Build history of the part. All positions in model axes, mm. Face numbers are marked on the shaded views. Coordinates: 2 decimals unless noted, no trailing zeros. Loops run counter-clockwise (first coordinate to the right, second up) from the corner with the lowest first, then second, coordinate; pieces in that order, holes last.
(1) Flat gauge pins, fed straight in: P1, Ø1, axis at x = -1, y = -1.5, coming from the -Z side; P2, Ø1.5, axis at y = 1, z = 2.5, coming from the +X side; P3, Ø0.7, axis at x = 0, z = -2, coming from the -Y side. Where does each tip first touch, or does it go through?
(2) Wall check: L1, parallel to Y at x = -0.75, z = 10.25; L2, parallel to X at y = 0.1, z = 15.5; L3, parallel to X at y = -1.3, z = 11. Give the ranges that are in metal, low to high.
(3) Two-plate mould, pull along X, no slides. Class the marked faces 1, 2 and 3: pulls with the +X half, pulls with the -X half, needs draft (parallel to the pull), parting line crosses it, or undercut.
(4) Slice it at A-A (z = 5.5). Give the cut face in (x, y).
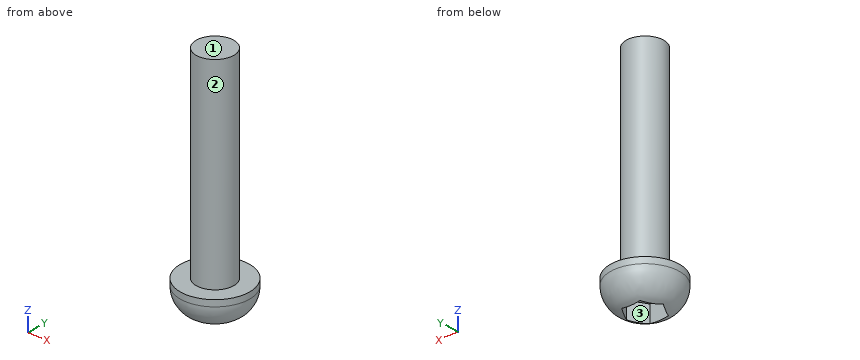
Autodesk Inventor part; units mm, degrees
ref_plane "YZ Plane" through (0, 0, 0) normal (1, 0, 0) x (0, 1, 0)
ref_plane "XZ Plane" through (0, 0, 0) normal (0, 1, 0) x (-1, 0, 0)
ref_plane "XY Plane" through (0, 0, 0) normal (0, 0, 1) x (1, 0, 0)
sketch "Boceto1" plane through (0, 0, 0) normal (0, 0, 1) x (1, 0, 0)
  circle A0 centre (0, 0) radius 1.5
  circle A1 centre (0, 0) radius 2.75
  dimension "d0" = 3
  dimension "d1" = 5.5
extrude "Extrusión1" add sketch "Boceto1" along normal blind 16 contours A0
extrude "Extrusión2" add sketch "Boceto1" against normal blind 2.5 contours A0 | A1
sketch "Boceto2" plane through (0, 0, -2.5) normal (0, 0, -1) x (-1, 0, 0)
  line L0 (1.5, 0) -> (0.75, -1.299)
  line L1 (0.75, -1.299) -> (-0.75, -1.299)
  line L2 (-0.75, -1.299) -> (-1.5, 0)
  line L3 (-1.5, 0) -> (-0.75, 1.299)
  line L4 (-0.75, 1.299) -> (0.75, 1.299)
  line L5 (0.75, 1.299) -> (1.5, 0)
  point P0 (0, 0)
  point P1 (0, 0)
  dimension "d6" = 3
fillet "Empalme1" radius 2 1 edges at (-2.75, 0, -2.5)
extrude "Extrusión4" cut sketch "Boceto2" against normal blind 1.5
thread "Rosca1"
properties part number "tonrilloM3x16mm" material "Acero inoxidable, 440C"
Response values:
1. P1: stops at z = -2.4
1. P2: stops at x = 1.48
1. P3: stops at y = -2.39
2. L1: y = -1.3 to 1.3
2. L2: x = -1.5 to 1.5
2. L3: x = -0.75 to 0.75
3. face 1: needs draft
3. face 2: parting line crosses it
3. face 3: undercut
4. outline: circle Ø3 at (0, 0)
